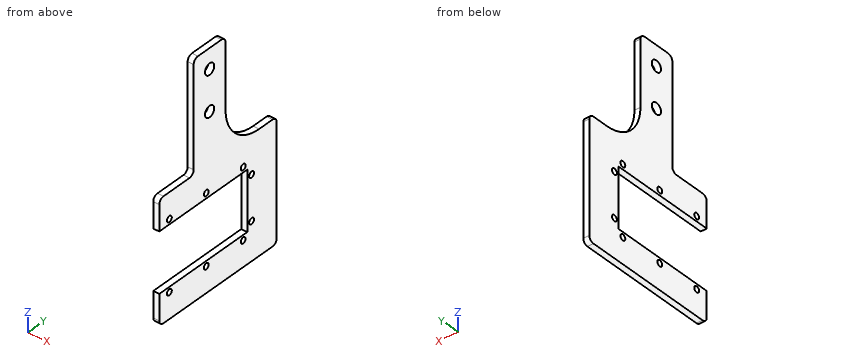
```python
from build123d import *

# Parameters (mm, degrees)
BOSS_EXTRUDE2_DEPTH        = 1.5
SKETCH11_W                 = 70
SKETCH11_H                 = 19
BOSS_EXTRUDE3_DEPTH        = 1.5
M5_CLEARANCE_HOLE1_D       = 5.5
FILLET1_R                  = 2.5
FILLET2_R                  = 2.5
M2_5_CLEARANCE_HOLE1_D     = 2.9
M2_5_CLEARANCE_HOLE1_DEPTH = 3
FILLET3_R                  = 20


with BuildPart() as part:
    # Sketch8 → Boss-Extrude2 (new, symmetric)
    with BuildSketch(Plane(origin=(0, 0, 0), x_dir=(0, 0, -1), z_dir=(1, 0, 0))):
        Polygon((30, 60), (-30, 60), (-30, -10), (-14.75, -10), (-14.75, 42.45), (14.75, 42.45), (14.75, -10), (30, -10), align=None)
    extrude(amount=BOSS_EXTRUDE2_DEPTH, both=True)

    # Sketch11 → Boss-Extrude3 (add, symmetric)
    with BuildSketch(Plane(origin=(0, 0, 0), x_dir=(0, 0, -1), z_dir=(1, 0, 0))):
        with Locations((-49.75, 20)):
            Rectangle(SKETCH11_W, SKETCH11_H)
    extrude(amount=BOSS_EXTRUDE3_DEPTH, both=True)

    # M5 Clearance Hole1 (through all)
    with Locations(Plane(origin=(1.5, 0, 0), x_dir=(0, 0, -1), z_dir=(1, 0, 0))):
        with Locations((-74.75, 20), (-54.75, 20)):
            Hole(M5_CLEARANCE_HOLE1_D / 2)

    # Fillet1
    fillet1_edges = [part.edges().sort_by_distance(p)[0] for p in [
        (0, 10.5, 84.75),
        (0, 29.5, 84.75),
    ]]
    fillet(fillet1_edges, radius=FILLET1_R)

    # Fillet2
    fillet2_edges = [part.edges().sort_by_distance(p)[0] for p in [
        (0, -10, -30),
        (0, -10, 30),
        (0, 60, 30),
        (0, 60, -30),
        (0, 10.5, 30),
    ]]
    fillet(fillet2_edges, radius=FILLET2_R)

    # M2.5 Clearance Hole1
    with Locations(Plane(origin=(1.5, 0, 0), x_dir=(0, 0, -1), z_dir=(1, 0, 0))):
        with Locations((17.3, 40), (79.72833177, 74.743551237), (17.3, 18), (17.3, -4), (-17.3, -4), (-17.3, 18), (-17.3, 40), (-11, 45), (11, 45)):
            Hole(M2_5_CLEARANCE_HOLE1_D / 2, depth=M2_5_CLEARANCE_HOLE1_DEPTH)

    # Fillet3
    fillet3_edges = [part.edges().sort_by_distance(p)[0] for p in [
        (0, 29.5, 30),
    ]]
    fillet(fillet3_edges, radius=FILLET3_R)


solid = part.part
```
Could you check a few things on this model? Use its own coordinates, in mm. Give positions to 0.01 mm unless a question says otherwise; leave off trailing zeros. Loops run counter-clockwise (first coordinate to the right, second up) from the corner with the lowest first, then second, coordinate; pieces in that order, holes last. Notation, with made-up numbers: (-4, 3.25) - (2, 3.25) arc R26 cw to (2, 20.25) - close; hole circle Ø2 at (88, -30.5). An arc over 180 degrees is marked (long way). Answer in a Markdown table with one row per item. Add a question column.
Q1. Please list where these lines run through material, in increasing order: L1, parallel to Y at x = 0.3, z = 17.3; L2, parallel to Z at x = -1.25, y = 8; L3, parallel to Y at x = 0.3, z = -11. Write a range as from..to.
Q2. For pin 1 (12 mm diameter, centred on y = 3, z = 54, fed in from +X); pin 2 (0.9 mm diameter, centred on x = 0, z = 68.5, fed in from +Y); pin 3 (1.5 mm diameter, centred on x = -1, z = 49, fed in from +Y); pin 4 (1.5 mm diameter, centred on x = 0.5, y = 54, fed in from +Z), each with a flat end and sliding along its axis, tell me the tip position at first contact or that it passes through.
Q3. If we section it at A-A (y = -4): List the corners of the cut face in (x, z) for me, plus the area to 3 significant figures.
Q4. If we section it at D-D (y = 6.5): List the corners of the cut face in (x, z) for me.
Q5. If we section it at B-B (z = 74.75): List the corners of the cut face in (x, y) for me.
Q6. If we section it at C-C (x = 0.25): State how many separate pieces and enclosed holes the cut face has, plus the area to 3 significant figures.
The answers:
| question | item | result |
|---|---|---|
| 1 | L1 | y = -10..-5.45, -2.55..16.55, 19.45..38.55, 41.45..60 |
| 1 | L2 | z = -30..-14.75, 14.75..30 |
| 1 | L3 | y = 42.45..43.55, 46.45..60 |
| 2 | pin 1 | passes through |
| 2 | pin 2 | stops at y = 29.5 |
| 2 | pin 3 | stops at y = 29.58 |
| 2 | pin 4 | stops at z = 30 |
| 3 | outline | (-1.5, -30) - (1.5, -30) - (1.5, -18.75) - (-1.5, -18.75) - close; (-1.5, -15.85) - (1.5, -15.85) - (1.5, -14.75) - (-1.5, -14.75) - close; (-1.5, 14.75) - (1.5, 14.75) - (1.5, 15.85) - (-1.5, 15.85) - close; (-1.5, 18.75) - (1.5, 18.75) - (1.5, 30) - (-1.5, 30) - close |
| 3 | area | 74.1 mm^2 |
| 4 | outline | (-1.5, -30) - (1.5, -30) - (1.5, -14.75) - (-1.5, -14.75) - close; (-1.5, 14.75) - (1.5, 14.75) - (1.5, 30) - (-1.5, 30) - close |
| 5 | outline | (-1.5, 10.5) - (1.5, 10.5) - (1.5, 17.25) - (-1.5, 17.25) - close; (-1.5, 22.75) - (1.5, 22.75) - (1.5, 29.5) - (-1.5, 29.5) - close |
| 6 | separate pieces | 1 |
| 6 | enclosed holes | 10 |
| 6 | area | 3,670 mm^2 |
